Print and shaded views of the part. All mm, measured from the part's lowest x, y and z. Coordinates: 2 decimals unless noted, no trailing zeros. Loops run counter-clockwise (first coordinate to the right, second up) from the corner with the lowest first, then second, coordinate; pieces in that order, holes last.
1) Pin check, flat tips, straight feed: pin 1 Ø5 at (y, z) = (8, 94.5) entering from +X; pin 2 Ø2 at (x, y) = (72, 4) entering from -Z; pin 3 Ø2 at (x, y) = (46.5, 6.5) entering from -Z; pin 4 Ø2 at (x, y) = (70, 4) entering from +Z. Stop position of each tip, or through.
2) Saw through at B-B, the plane z = 151.5. Write the cut outline in (x, y).
3) Wall check: line 1 along Z through (x, y) = (70.5, 2); line 2 along Z through (x, y) = (57, 6.5); line 3 along X through (y, z) = (1, 74). Give the ranges that are in metal, low to high.
4) Saw through at D-D, the plane x = 12. Write the cut outline in (y, z).
5) Saw through at A-A, the plane x = 57. Write the cut outline in (y, z), and give its area (4 significant figures).
6) Saw through at C-C, the plane y = 5.5. Write the cut outline in (x, z).
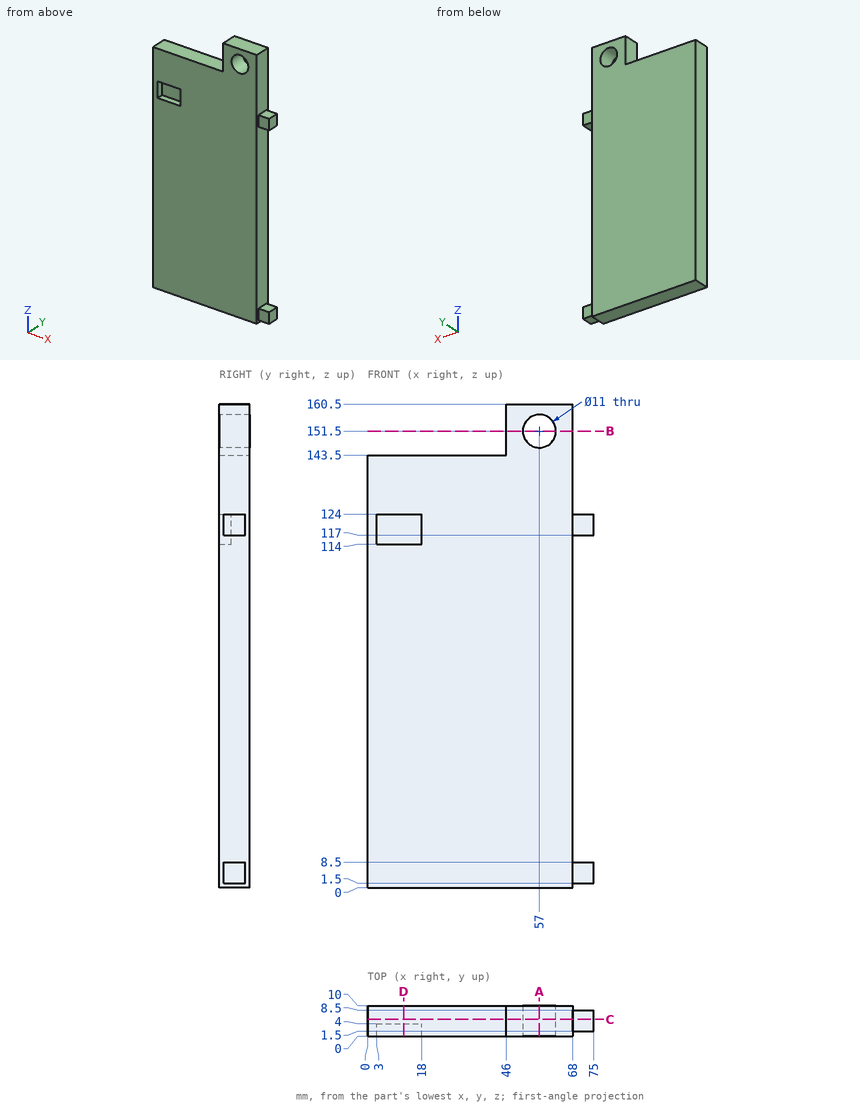
Data:
1. pin 1: stops at x = 68
1. pin 2: stops at z = 1.5
1. pin 3: stops at z = 0
1. pin 4: stops at z = 124
2. outline: (46, 0) - (51.5, 0) - (51.5, 10) - (46, 10) - close; (62.5, 0) - (68, 0) - (68, 10) - (62.5, 10) - close
3. line 1: z = 1.5 to 8.5, 117 to 124
3. line 2: z = 0 to 146, 157 to 160.5
3. line 3: x = 0 to 68
4. outline: (0, 0) - (10, 0) - (10, 143.5) - (0, 143.5) - (0, 124) - (4, 124) - (4, 114) - (0, 114) - close
5. outline: (0, 0) - (10, 0) - (10, 146) - (0, 146) - close; (0, 157) - (10, 157) - (10, 160.5) - (0, 160.5) - close
5. area: 1,495 mm2
6. outline: (0, 0) - (68, 0) - (68, 1.5) - (75, 1.5) - (75, 8.5) - (68, 8.5) - (68, 117) - (75, 117) - (75, 124) - (68, 124) - (68, 160.5) - (46, 160.5) - (46, 143.5) - (0, 143.5) - close; hole circle Ø11 at (57, 151.5)
